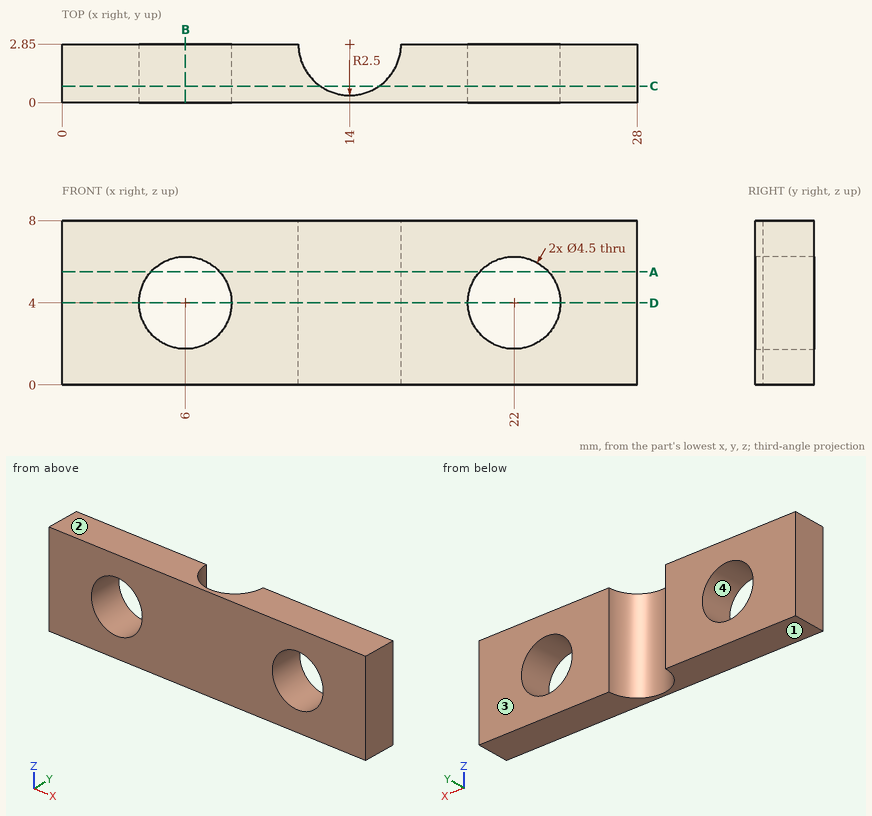
For this review, use the dimensioned drawing (mm, ordinates from the lowest corner) and the shaded views. Coordinates: 2 decimals unless noted, no trailing zeros. Write each loop counter-clockwise with the first axis right and the second up, starting at its lowest first coordinate (ties: lowest second). Pieces come first, ordered by that corner, then holes. Notation, with made-up numbers: (-2, 38.25) -> (13, 38.25) arc R20 ccw to (13, 50.25) -> close; hole circle Ø1 at (86, 69). An arc over 180 degrees is marked (long way). Put each result on its own line as item: value.
Q1. The part is to be moulded in two halves that separate along Z. For the marked faces 1, 2, 3 and 4, say which applies: +Z half, -Z half, draft (parallel to the pull), parting line (faces both ways), or undercut.
From the geometry:
face 1: -Z half
face 2: +Z half
face 3: draft
face 4: undercut
Q2. Wall thickness on L1, parallel to X at y = 2.2, z = 3.25; L2, parallel to X at y = 1.75, z = 4 (3 decimals); L3, parallel to X at y = 1.35, z = 6.5: over which ranges is each line inside the solid? List them lowest first.
From the geometry:
L1: x = 0 to 3.88, 8.12 to 11.59, 16.41 to 19.88, 24.12 to 28
L2: x = 0 to 3.75, 8.25 to 11.755, 16.245 to 19.75, 24.25 to 28
L3: x = 0 to 12, 16 to 28
Q3. Take a section at B-B, the plane x = 6. State the section outline as (y, z) points, then the cut area to 4 significant figures.
From the geometry:
outline: (0, 0) -> (2.85, 0) -> (2.85, 1.75) -> (0, 1.75) -> close; (0, 6.25) -> (2.85, 6.25) -> (2.85, 8) -> (0, 8) -> close
area: 9.975 mm2
Q4. Take a section at D-D, the plane z = 4. State the section outline as (x, y) points, then the cut area to 3 significant figures.
From the geometry:
outline: (0, 0) -> (3.75, 0) -> (3.75, 2.85) -> (0, 2.85) -> close; (8.25, 0) -> (19.75, 0) -> (19.75, 2.85) -> (16.5, 2.85) arc R2.5 cw to (11.5, 2.85) -> (8.25, 2.85) -> close; (24.25, 0) -> (28, 0) -> (28, 2.85) -> (24.25, 2.85) -> close
area: 44.3 mm2
Q5. Take a section at A-A, the plane z = 5.5. State the section outline as (x, y) points, then the cut area to 3 significant figures.
From the geometry:
outline: (0, 0) -> (4.32, 0) -> (4.32, 2.85) -> (0, 2.85) -> close; (7.68, 0) -> (20.32, 0) -> (20.32, 2.85) -> (16.5, 2.85) arc R2.5 cw to (11.5, 2.85) -> (7.68, 2.85) -> close; (23.68, 0) -> (28, 0) -> (28, 2.85) -> (23.68, 2.85) -> close
area: 50.9 mm2
Q6. Take a section at C-C, the plane y = 0.8. State the section outline as (x, z) points, then the cut area to 3 significant figures.
From the geometry:
outline: (0, 0) -> (12.57, 0) -> (12.57, 8) -> (0, 8) -> close; (15.43, 0) -> (28, 0) -> (28, 8) -> (15.43, 8) -> close; hole circle Ø4.5 at (6, 4); hole circle Ø4.5 at (22, 4)
area: 169 mm2
Q7. Clearance check with flat-ended pins moving along their axes: pin 1 Ø2 at (x, z) = (14.5, 2) entering from +Y; pin 2 Ø4 at (x, z) = (22, 4) entering from -Y. State where each tip first meets the part, or that it passes through.
From the geometry:
pin 1: stops at y = 0.85
pin 2: passes through
